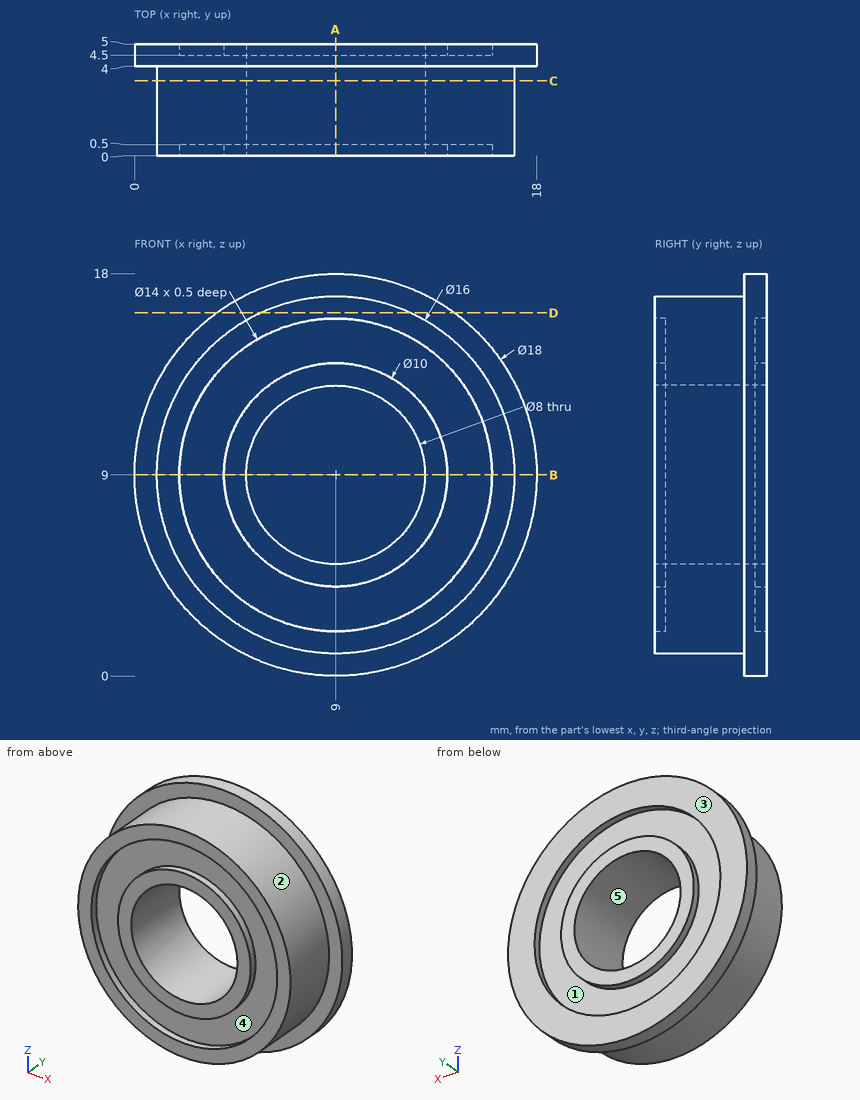
Verification items for this drawing (mm, ordinates from the low corner). A direction names the side the tool comes from. Give positions to 0.01 mm unless a question says otherwise; leave off trailing zeros. Loops run counter-clockwise (first coordinate to the right, second up) from the corner with the lowest first, then second, coordinate; pieces in that order, holes last. Notation, with made-up numbers: M 72.5,48.25 L 123.5,48.25 A25 cw 123.5,75.25 Z; hole C -2,-0.5 d4. An arc over 180 degrees is marked long. Answer in a Markdown table with one row per item.
1) Cross-section at B-B (z = 9). Enter the section's corners in (x, y), plus the area to 3 significant figures.
Solutions:
| item | result |
|---|---|
| outline | M 0,4 L 1,4 L 1,0 L 2,0 L 2,0.5 L 4,0.5 L 4,0 L 5,0 L 5,5 L 4,5 L 4,4.5 L 2,4.5 L 2,5 L 0,5 Z; M 13,0 L 14,0 L 14,0.5 L 16,0.5 L 16,0 L 17,0 L 17,4 L 18,4 L 18,5 L 16,5 L 16,4.5 L 14,4.5 L 14,5 L 13,5 Z |
| area | 38.0 mm^2 |
2) Cross-section at C-C (y = 3.35). Enter the section's corners in (x, z).
Solutions:
| item | result |
|---|---|
| outline | C 9,9 d16; hole C 9,9 d8 |
3) Mould release check, pull along X, two halves, no side actions. Record for the marked faces 1, 2 and 3: released by +X, released by -X, zero draft, split by the parting line, or undercut.
Solutions:
| item | result |
|---|---|
| face 1 | undercut |
| face 2 | split by the parting line |
| face 3 | zero draft |
4) Thickness scan on line 1 (X direction, y = 0.25, z = 9); line 2 (X direction, y = 4.9, z = 9); line 3 (Z direction, x = 12, y = 0.25). Record the ranges inside material, lowest first.
Solutions:
| item | result |
|---|---|
| line 1 | x = 1 to 2, 4 to 5, 13 to 14, 16 to 17 |
| line 2 | x = 0 to 2, 4 to 5, 13 to 14, 16 to 18 |
| line 3 | z = 1.58 to 2.68, 5 to 6.35, 11.65 to 13, 15.32 to 16.42 |
5) Depth check by flat-ended pin: pin 1 (3 mm diameter, centred on x = 3.5, y = 2, fed in from -Z); pin 2 (1 mm diameter, centred on x = 11, y = 3, fed in from -Z); pin 3 (6.5 mm diameter, centred on x = 9, z = 9, fed in from +Y); pin 4 (3 mm diameter, centred on y = 2, z = 11, fed in from -X). Enter the tip coordinate at first touch or a pass-through.
Solutions:
| item | result |
|---|---|
| pin 1 | stops at z = 2.07 |
| pin 2 | stops at z = 1.14 |
| pin 3 | passes through |
| pin 4 | stops at x = 1.02 |
6) Cross-section at A-A (x = 9). Enter the section's corners in (y, z).
Solutions:
| item | result |
|---|---|
| outline | M 0,1 L 4,1 L 4,0 L 5,0 L 5,2 L 4.5,2 L 4.5,4 L 5,4 L 5,5 L 0,5 L 0,4 L 0.5,4 L 0.5,2 L 0,2 Z; M 0,13 L 5,13 L 5,14 L 4.5,14 L 4.5,16 L 5,16 L 5,18 L 4,18 L 4,17 L 0,17 L 0,16 L 0.5,16 L 0.5,14 L 0,14 Z |
7) Tool access check on the marked faces 4 and 5. Record the directions out of +Z, -Z, +X, -X, +Y, -Y that give a thin tool (end or side, any length) a straight path to the whole face; none if there is none.
Solutions:
| item | result |
|---|---|
| face 4 | -Y |
| face 5 | +Y, -Y |
8) Cross-section at D-D (z = 16.25). Enter the section's corners in (x, y).
Solutions:
| item | result |
|---|---|
| outline | M 3.67,4 L 5.62,4 L 5.62,0 L 12.38,0 L 12.38,4 L 14.33,4 L 14.33,5 L 3.67,5 Z |
